```python
from build123d import *

# Parameters (mm, degrees)
SKETCH009_W             = 120.6
SKETCH009_H             = 82.6
PAD006_DEPTH            = 1.6
SKETCH010_W             = 120.6
SKETCH010_H             = 82.6
SKETCH010_W_2           = 118.6
SKETCH010_H_2           = 80.6
PAD007_DEPTH            = 20.8
SKETCH011_W             = 11.5
SKETCH011_H             = 9
PAD008_DEPTH            = 14.8
SKETCH012_W             = 11.5
SKETCH012_H             = 2
PAD009_DEPTH            = 22.5
SKETCH014_R             = 1.75
POCKET004_DEPTH         = 1.6
SKETCH020_W             = 11.5
SKETCH020_H             = 20
PAD013_DEPTH            = 22.1
BODY003_PLACEMENT_ANGLE = 180


with BuildPart() as part:
    # Sketch009 → Pad006 (new body)
    with BuildSketch(Plane.XY):
        Rectangle(SKETCH009_W, SKETCH009_H)
    extrude(amount=PAD006_DEPTH)

    # Sketch010 → Pad007 (join)
    with BuildSketch(Plane.XY):
        Rectangle(SKETCH010_W, SKETCH010_H)
        Rectangle(SKETCH010_W_2, SKETCH010_H_2, mode=Mode.SUBTRACT)
    extrude(amount=PAD007_DEPTH)

    # Sketch011 → Pad008 (join)
    with BuildSketch(Plane.XY):
        with Locations((-51.95, -27.2)):
            Rectangle(SKETCH011_W, SKETCH011_H)
    extrude(amount=PAD008_DEPTH)

    # Sketch012 → Pad009 (join)
    with BuildSketch(Plane.XY):
        with Locations((-51.95, -21.7)):
            Rectangle(SKETCH012_W, SKETCH012_H)
    extrude(amount=PAD009_DEPTH)

    # Sketch014 → Pocket004 (cut)
    with BuildSketch(Plane.XY):
        with Locations((-55, 36)):
            Circle(SKETCH014_R)
        with Locations((1, 36)):
            Circle(SKETCH014_R)
        with Locations((55, 36)):
            Circle(SKETCH014_R)
        with Locations((55, -36)):
            Circle(SKETCH014_R)
        with Locations((1, -36)):
            Circle(SKETCH014_R)
        with Locations((-55, -36)):
            Circle(SKETCH014_R)
    extrude(amount=POCKET004_DEPTH, mode=Mode.SUBTRACT)

    # Sketch020 → Pad013 (join)
    with BuildSketch(Plane.XY):
        with Locations((-51.95, 21.7)):
            Rectangle(SKETCH020_W, SKETCH020_H)
    extrude(amount=PAD013_DEPTH)


with BuildPart() as part_1:
    # Body003 placement: moved
    add(part.part.moved(Location((0, 0, 57.9))).rotate(Axis((0, 0, 57.9), (1, 0, 0)), BODY003_PLACEMENT_ANGLE))


solid = part_1.part
```
Geometry check sheet. Reference: the model listing, model coordinates, mm. A direction names the side the tool comes from. Round coordinates to 2 decimals unless told otherwise and drop trailing zeros. Loops run counter-clockwise (first coordinate to the right, second up) from the corner with the lowest first, then second, coordinate; pieces in that order, holes last. Notation, with made-up numbers: (10, 3.5) - (55, 3.5) arc R27 ccw to (55, 20.5) - close; hole circle Ø10 at (25, 82). An arc over 180 degrees is marked (long way). Write item = value, one per line. Start each with the question number.
1. Set-up check for faces 4 (the face through (-59.3, 1, 47)), 5 (the face through (-52, -22, 35.8)), 6 (the face through (-53.383, 36.67, 57.111)): record each of +Z, -Z, +X, -X, +Y, -Y from which the full face is reachable in a straight line by a thin tool's end or side.
2. Section check D-D on z = 50. Enter the section's corners in (x, y).
3. Thickness scan on line 1 (X direction, y = -36, z = 57); line 2 (Y direction, x = -55, z = 57.55); line 3 (X direction, y = 27.5, z = 54.25). Record the ranges inside material, lowest first.
4. Section check A-A on z = 41. Enter the section's corners in (x, y), then the cut area to 3 significant figures.
5. Depth check by flat-ended pin: pin 1 (4.5 mm diameter, centred on x = 55, y = 36, fed in from -Z); pin 2 (6 mm diameter, centred on x = -54.5, y = -26, fed in from -Z). Enter the tip coordinate at first touch or a pass-through.
6. Section check C-C on y = 36. Enter the section's corners in (x, z).
7. Mould release check, pull along Y, two halves, no side actions. Record for faces 1 (the face through (-1, 40.3, 47)), 2 (the face through (-1, -1, 57.9)), 3 (the face through (-1, -41.3, 48)): released by +Y, released by -Y, zero draft, split by the parting line, or undercut.
8. Section check B-B on x = -55. Enter the section's corners in (y, z).
Working result:
q1.face_4 = -Z
q1.face_5 = -Z, +X, -X, -Y
q1.face_6 = +Z, -Z
q2.outline = (-60.3, -41.3) - (60.3, -41.3) - (60.3, 41.3) - (-60.3, 41.3) - close; (-57.7, -31.7) - (-46.2, -31.7) - (-46.2, -11.7) - (-57.7, -11.7) - close; (-57.7, 20.7) - (-46.2, 20.7) - (-46.2, 31.7) - (-57.7, 31.7) - close; hole (-59.3, -40.3) - (59.3, -40.3) - (59.3, 40.3) - (-59.3, 40.3) - close
q3.line_1 = -60.3 to -56.75, -53.25 to -0.75, 2.75 to 53.25, 56.75 to 60.3
q3.line_2 = -41.3 to -37.75, -34.25 to 34.25, 37.75 to 41.3
q3.line_3 = -60.3 to -59.3, -57.7 to -46.2, 59.3 to 60.3
q4.outline = (-60.3, -41.3) - (60.3, -41.3) - (60.3, 41.3) - (-60.3, 41.3) - close; (-57.7, -31.7) - (-46.2, -31.7) - (-46.2, -11.7) - (-57.7, -11.7) - close; (-57.7, 20.7) - (-46.2, 20.7) - (-46.2, 22.7) - (-57.7, 22.7) - close; hole (-59.3, -40.3) - (59.3, -40.3) - (59.3, 40.3) - (-59.3, 40.3) - close
q4.area = 655 mm^2
q5.pin_1 = 56.3
q5.pin_2 = 35.8
q6.outline = (-60.3, 37.1) - (-59.3, 37.1) - (-59.3, 56.3) - (-56.75, 56.3) - (-56.75, 57.9) - (-60.3, 57.9) - close; (-53.25, 56.3) - (-0.75, 56.3) - (-0.75, 57.9) - (-53.25, 57.9) - close; (2.75, 56.3) - (53.25, 56.3) - (53.25, 57.9) - (2.75, 57.9) - close; (56.75, 56.3) - (59.3, 56.3) - (59.3, 37.1) - (60.3, 37.1) - (60.3, 57.9) - (56.75, 57.9) - close
q7.face_1 = undercut
q7.face_2 = zero draft
q7.face_3 = released by -Y
q8.outline = (-41.3, 37.1) - (-40.3, 37.1) - (-40.3, 56.3) - (-37.75, 56.3) - (-37.75, 57.9) - (-41.3, 57.9) - close; (-34.25, 56.3) - (-31.7, 56.3) - (-31.7, 35.8) - (-11.7, 35.8) - (-11.7, 56.3) - (20.7, 56.3) - (20.7, 35.4) - (22.7, 35.4) - (22.7, 43.1) - (31.7, 43.1) - (31.7, 56.3) - (34.25, 56.3) - (34.25, 57.9) - (-34.25, 57.9) - close; (37.75, 56.3) - (40.3, 56.3) - (40.3, 37.1) - (41.3, 37.1) - (41.3, 57.9) - (37.75, 57.9) - close
